```python
from build123d import *

# Parameters (mm, degrees)
SKETCH1_W               = 100
SKETCH1_H               = 60
BOSS_EXTRUDE4_DEPTH     = 10
CUT_EXTRUDE1_DEPTH      = 105.880884817
CUT_EXTRUDE1_DEPTH_BACK = 100
SKETCH3_W               = 59.99788365
SKETCH3_H               = 10
BOSS_EXTRUDE5_DEPTH     = 100
SKETCH4_W               = 100
SKETCH4_H               = 5
CUT_EXTRUDE2_DEPTH      = 60
SKETCH5_W               = 100
SKETCH5_H               = 2.5
CUT_EXTRUDE3_DEPTH      = 60


with BuildPart() as part:
    # Sketch1 → Boss-Extrude4 (new body)
    with BuildSketch(Plane(origin=(0, 0, 0), x_dir=(1, 0, 0), z_dir=(0, 1, 0))):
        Rectangle(SKETCH1_W, SKETCH1_H)
    extrude(amount=BOSS_EXTRUDE4_DEPTH)

    # Sketch2 → Cut-Extrude1 (cut, two sides: drawn at the far end of the back side and taken through both)
    with BuildSketch(Plane(origin=(50, 0, 0), x_dir=(0, 0, -1), z_dir=(1, 0, 0)).offset(-CUT_EXTRUDE1_DEPTH_BACK)):
        with BuildLine():
            Line((-135.324200485, 88.993150364), (-30, 10))
            ThreePointArc((-30, 10), (0, 0), (30, 10))
            Line((30, 10), (135.324200485, 88.993150364))
            Line((135.324200485, 88.993150364), (135.324200485, 352.303651576))
            Line((135.324200485, 352.303651576), (-135.324200485, 352.303651576))
            Line((-135.324200485, 352.303651576), (-135.324200485, 88.993150364))
        make_face()
    extrude(amount=CUT_EXTRUDE1_DEPTH + CUT_EXTRUDE1_DEPTH_BACK, mode=Mode.SUBTRACT)


with BuildPart() as cut_extrude1_piece_1:
    # of the separate pieces the step leaves, piece 1, a body of its own (cut_extrude1_pieces)
    add(part.part.solids().sort_by_distance((50, 0, 30))[0])



with BuildPart() as cut_extrude1_piece_2:
    # of the separate pieces the step leaves, piece 2, a body of its own (cut_extrude1_pieces)
    add(part.part.solids().sort_by_distance((50, 0, -30))[0])


with BuildPart() as cut_extrude1_piece_1_1:
    add(cut_extrude1_piece_1.part)

    add(cut_extrude1_piece_2.part)  # Boss-Extrude5 merges Cut-Extrude1 piece 2
    # Sketch3 → Boss-Extrude5 (add)
    with BuildSketch(Plane(origin=(50, 0, 0), x_dir=(0, 0, -1), z_dir=(1, 0, 0))):
        with Locations((-0.001058175, -5)):
            Rectangle(SKETCH3_W, SKETCH3_H)
    extrude(amount=-BOSS_EXTRUDE5_DEPTH)

    # Sketch4 → Cut-Extrude2 (cut)
    with BuildSketch(Plane(origin=(0, 0, -29.99788365), x_dir=(-1, 0, 0), z_dir=(0, 0, -1))):
        with Locations((0, -7.5)):
            Rectangle(SKETCH4_W, SKETCH4_H)
    extrude(amount=-CUT_EXTRUDE2_DEPTH, mode=Mode.SUBTRACT)

    # Sketch5 → Cut-Extrude3 (cut)
    with BuildSketch(Plane(origin=(0, 0, -29.99788365), x_dir=(-1, 0, 0), z_dir=(0, 0, -1))):
        with Locations((0, -3.75)):
            Rectangle(SKETCH5_W, SKETCH5_H)
    extrude(amount=-CUT_EXTRUDE3_DEPTH, mode=Mode.SUBTRACT)


solid = cut_extrude1_piece_1_1.part
```
Can you work these out from the model? Positions are in its coordinate system, mm. Coordinates: 2 decimals unless noted, no trailing zeros. Loops run counter-clockwise (first coordinate to the right, second up) from the corner with the lowest first, then second, coordinate; pieces in that order, holes last.
Item 1: I'm going to push flat-ended pins straight in: pin 1 (2 mm diameter, centred on x = -10, y = -1, fed in from -Z); pin 2 (6 mm diameter, centred on x = 0.5, z = 18.5, fed in from +Y); pin 3 (1 mm diameter, centred on x = -22, z = -0.5, fed in from +Y); pin 4 (3 mm diameter, centred on y = 3, z = -1.5, fed in from +X). Where does each tip first touch, or does it pass through?
Answers below:
pin 1: stops at z = -30
pin 2: stops at y = 4.86
pin 3: stops at y = 0.01
pin 4: passes through
Item 2: Suppose I cut it at A-A (y = 8.75). Please give me the cut outline in (x, z).
Answers below:
outline: (-50, -30) - (50, -30) - (50, -28.26) - (-50, -28.26) - close; (-50, 28.26) - (50, 28.26) - (50, 30) - (-50, 30) - close
Item 3: If we mould it in two halves opening along Z, with no side actions, what happens to faces 1 (the face through (1, -1, -29.998)), 2 (the face through (1, 4, 30)), 3 (the face through (50, -0.3, 0.4)), 4 (the face through (-1, 0, 0))? For each: released by +Z, released by -Z, zero draft, split by the parting line, or undercut.
Answers below:
face 1: released by -Z
face 2: released by +Z
face 3: zero draft
face 4: undercut
Item 4: Suppose I cut it at B-B (z = -1). Please give me the cut outline in (x, y).
Answers below:
outline: (-50, -2.5) - (50, -2.5) - (50, 0.01) - (-50, 0.01) - close
Item 5: Suppose I cut it at D-D (z = -14). Please give me the cut outline in (x, y).
Answers below:
outline: (-50, -2.5) - (50, -2.5) - (50, 2) - (-50, 2) - close
Item 6: Please list where these lines run through material, in increasing order: L1, parallel to Z at x = -31.5, y = 8.5; L2, parallel to Z at x = 17.5, y = 4.5; L3, parallel to Y at x = -40.5, z = 0.5.
Answers below:
L1: z = -30 to -27.89, 27.89 to 30
L2: z = -30 to -20.73, 20.73 to 30
L3: y = -2.5 to 0
